```python
from build123d import *

# Parameters (mm, degrees)
F1_DEPTH = 9.5


with BuildPart() as f1:
    # F0 (on Front) → F1 (new body, symmetric)
    with BuildSketch(Plane.XZ):
        Polygon((-275, 75), (-275, -275), (275, -275), (275, 275), (-75, 275), align=None)
        Polygon((35, -260), (-260, -260), (-260, -130), (-267.5, -130), (-267.5, -115), (-260, -115), (-260, 68.7867965644), (-68.7867965644, 260), (115, 260), (115, 267.5), (130, 267.5), (130, 260), (260, 260), (260, -35), (267.5, -35), (267.5, -50), (260, -50), (260, -260), (50, -260), (50, -267.5), (35, -267.5), align=None, mode=Mode.SUBTRACT)
    extrude(amount=F1_DEPTH, both=True)


solid = f1.part
```
Geometry: final body of the model. Coordinates: model frame, mm. A direction names the side the tool comes from. Round coordinates to 2 decimals unless told otherwise and drop trailing zeros. Order: outer loops, then holes, each group sorted by start corner. A loop starts at its lowest first (then second) coordinate and runs counter-clockwise, first axis right, second up. Notation, with made-up numbers: (-34, 61.25) - (1, 61.25) arc R8 cw to (1, 68.25) - close; hole circle Ø2 at (43.25, 36.5). An arc over 180 degrees is marked (long way). Use CSV: the item, a comma, the result in double quotes. Start each with the question number.
Q1. Section query C-C (y = -4.25). Return loops of the section in (x, z), and give its area (3 significant figures).
Q2. Material intervals for line 1 along Z through (x, y) = (-26, 2); line 2 along X through (y, z) = (0.25, 167), sorted ascending. Write a range as from..to.
Q3. Section query A-A (z = -100). Return loops of the section in (x, y), and give its area (3 significant figures).
Q4. Mould query, pull axis X, two halves, no side actions, for faces 3 (the face through (19, 9.5, -264)), 4 (the face through (-174, 0, 176)), 5 (the face through (-260, 0, -24)), 6 (the face through (275, 0, -4)). Classes: +X half, -X half, draft (parallel to the pull), parting line (faces both ways), or undercut.
Q5. Access query for faces 1 (the face through (-260, 0, -196)), 2 (the face through (-4, 0, -275)). Directions: +Z, -Z, +X, -X, +Y, -Y. A direction counts if a zero-diameter tool reaches every point of the face in a straight line with its end or side. Return the directions, or none.
Q6. Section query B-B (x = -17.5). Return loops of the section in (y, z), and give its area (3 significant figures).
Result set:
1,outline,"(-275, -275) - (275, -275) - (275, 275) - (-75, 275) - (-275, 75) - close; hole (-267.5, -130) - (-260, -130) - (-260, -260) - (35, -260) - (35, -267.5) - (50, -267.5) - (50, -260) - (260, -260) - (260, -50) - (267.5, -50) - (267.5, -35) - (260, -35) - (260, 260) - (130, 260) - (130, 267.5) - (115, 267.5) - (115, 260) - (-68.79, 260) - (-260, 68.79) - (-260, -115) - (-267.5, -115) - close"
1,area,"29,900 mm2"
2,line 1,"z = -275..-260, 260..275"
2,line 2,"x = -183..-161.79, 260..275"
3,outline,"(-275, -9.5) - (-260, -9.5) - (-260, 9.5) - (-275, 9.5) - close; (260, -9.5) - (275, -9.5) - (275, 9.5) - (260, 9.5) - close"
3,area,"570 mm2"
4,face 3,"draft"
4,face 4,"-X half"
4,face 5,"undercut"
4,face 6,"+X half"
5,face 1,"+Y, -Y"
5,face 2,"-Z, +X, -X, +Y, -Y"
6,outline,"(-9.5, -275) - (9.5, -275) - (9.5, -260) - (-9.5, -260) - close; (-9.5, 260) - (9.5, 260) - (9.5, 275) - (-9.5, 275) - close"
6,area,"570 mm2"
